```python
from build123d import *

# Parameters (mm, degrees)
BOSS_EXTRU_1_DEPTH      = 5
ENL_V_MAT_EXTRU_1_DEPTH = 3
ESQUISSE3_W             = 33.2
ESQUISSE3_H             = 3
ENL_V_MAT_EXTRU_2_DEPTH = 3
ESQUISSE4_W             = 5
ESQUISSE4_H             = 1
BOSS_EXTRU_2_DEPTH      = 0.48904
ESQUISSE5_W             = 5
ESQUISSE5_H             = 1
BOSS_EXTRU_3_DEPTH      = 0.48904
ESQUISSE6_W             = 5
ESQUISSE6_H             = 1
BOSS_EXTRU_4_DEPTH      = 0.48904


with BuildPart() as part:
    # Esquisse1 → Boss.-Extru.1 (new body)
    with BuildSketch(Plane(origin=(0, 0, 0), x_dir=(1, 0, 0), z_dir=(0, 1, 0))):
        with BuildLine():
            Line((2, 0), (36.2, 0))
            ThreePointArc((36.2, 0), (37.614213562, 0.585786438), (38.2, 2))
            Line((38.2, 2), (38.2, 25))
            ThreePointArc((38.2, 25), (37.614213562, 26.414213562), (36.2, 27))
            Line((36.2, 27), (2, 27))
            ThreePointArc((2, 27), (0.585786438, 26.414213562), (0, 25))
            Line((0, 25), (0, 2))
            ThreePointArc((0, 2), (0.585786438, 0.585786438), (2, 0))
        make_face()
    extrude(amount=BOSS_EXTRU_1_DEPTH)

    # Esquisse2 → Enlèv. mat.-Extru.1 (cut)
    with BuildSketch(Plane(origin=(0, 5, 0), x_dir=(1, 0, 0), z_dir=(0, 1, 0))):
        with BuildLine():
            Line((37.2, 2), (37.2, 25))
            ThreePointArc((37.2, 25), (36.907106781, 25.707106781), (36.2, 26))
            Line((36.2, 26), (2, 26))
            ThreePointArc((2, 26), (1.292893219, 25.707106781), (1, 25))
            Line((1, 25), (1, 2))
            ThreePointArc((1, 2), (1.292893219, 1.292893219), (2, 1))
            Line((2, 1), (36.2, 1))
            ThreePointArc((36.2, 1), (36.907106781, 1.292893219), (37.2, 2))
        make_face()
    extrude(amount=-ENL_V_MAT_EXTRU_1_DEPTH, mode=Mode.SUBTRACT)

    # Esquisse3 → Enlèv. mat.-Extru.2 (cut)
    with BuildSketch(Plane.XY):
        with Locations((19.1, 3.5)):
            Rectangle(ESQUISSE3_W, ESQUISSE3_H)
    extrude(amount=-ENL_V_MAT_EXTRU_2_DEPTH, mode=Mode.SUBTRACT)

    # Esquisse4 → Boss.-Extru.2 (add)
    with BuildSketch(Plane(origin=(1, 0, 0), x_dir=(0, 0, -1), z_dir=(1, 0, 0))):
        with Locations((13.5, 4.25)):
            Rectangle(ESQUISSE4_W, ESQUISSE4_H)
    extrude(amount=BOSS_EXTRU_2_DEPTH)

    # Esquisse5 → Boss.-Extru.3 (add)
    with BuildSketch(Plane.ZY.offset(-37.2)):
        with Locations((-13.5, 4.25)):
            Rectangle(ESQUISSE5_W, ESQUISSE5_H)
    extrude(amount=BOSS_EXTRU_3_DEPTH)

    # Esquisse6 → Boss.-Extru.4 (add)
    with BuildSketch(Plane.XY.offset(-26)):
        with Locations((9.75, 4.25)):
            Rectangle(ESQUISSE6_W, ESQUISSE6_H)
        with Locations((28.45, 4.25)):
            Rectangle(ESQUISSE6_W, ESQUISSE6_H)
    extrude(amount=BOSS_EXTRU_4_DEPTH)


solid = part.part
```
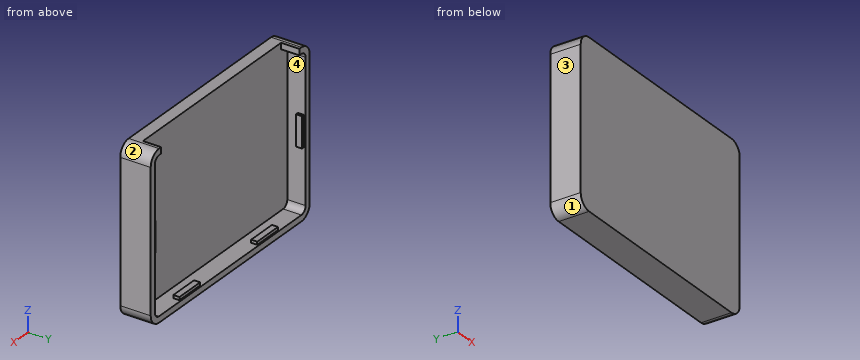
Could you check a few things on this model? Use its own coordinates, in mm. Face numbers are marked on the shaded views. Round coordinates to 2 decimals unless told otherwise and drop trailing zeros. Loops run counter-clockwise (first coordinate to the right, second up) from the corner with the lowest first, then second, coordinate; pieces in that order, holes last. Notation, with made-up numbers: (52, 76.25) - (91, 76.25) arc R28 ccw to (91, 95.25) - close; hole circle Ø11 at (-37, 1). An arc over 180 degrees is marked (long way). Answer as CSV lines item,"result".
1. I want a section at C-C on z = -5.5. List the corners of the cut face in (x, y) for me.
Filled in:
outline,"(0, 0) - (38.2, 0) - (38.2, 5) - (37.2, 5) - (37.2, 2) - (1, 2) - (1, 5) - (0, 5) - close"
2. I want a section at A-A on y = 3.35. List the corners of the cut face in (x, z) for me.
Filled in:
outline,"(0, -25) arc R2 ccw to (2, -27) - (36.2, -27) arc R2 ccw to (38.2, -25) - (38.2, -2) arc R2 ccw to (36.2, 0) - (35.7, 0) - (35.7, -1) - (36.2, -1) arc R1 cw to (37.2, -2) - (37.2, -25) arc R1 cw to (36.2, -26) - (2, -26) arc R1 cw to (1, -25) - (1, -2) arc R1 cw to (2, -1) - (2.5, -1) - (2.5, 0) - (2, 0) arc R2 ccw to (0, -2) - close"
3. We'd pull the mould along Z, two halves only. Please class the marked faces 1, 2, 3 and 4: +Z half, -Z half, draft (parallel to the pull), parting line (faces both ways), or undercut.
Filled in:
face 1,"-Z half"
face 2,"+Z half"
face 3,"draft"
face 4,"undercut"
4. For pin 1 Ø1.5 at (x, z) = (6, -13.5) entering from +Y; pin 2 Ø1 at (x, z) = (26, -15.5) entering from -Y; pin 3 Ø0.5 at (y, z) = (4, -26) entering from -X; pin 4 Ø0.5 at (x, y) = (37, 4.5) entering from -Z, each with a flat end and sliding along its axis, tell me the tip position at first contact or that it passes through.
Filled in:
pin 1,"stops at y = 2"
pin 2,"stops at y = 0"
pin 3,"stops at x = 0.15"
pin 4,"stops at z = -26.92"
5. I want a section at B-B on x = 27.5. List the corners of the cut face in (y, z) for me, then the cut area to 3 significant figures.
Filled in:
outline,"(0, -27) - (5, -27) - (5, -26) - (4.75, -26) - (4.75, -25.51) - (3.75, -25.51) - (3.75, -26) - (2, -26) - (2, 0) - (0, 0) - close"
area,"57.5 mm^2"
6. Please list where these lines run through material, in increasing order: line 1 along X through (y, z) = (4.8, -14.5); line 2 along Y through (x, z) = (18, -24.5); line 3 along Z through (x, y) = (9, 3.4). Write a range as [from, to].
Filled in:
line 1,"x = [0, 1], [37.2, 38.2]"
line 2,"y = [0, 2]"
line 3,"z = [-27, -26]"
7. I want a section at D-D on z = -11.75. List the corners of the cut face in (x, y) for me.
Filled in:
outline,"(0, 0) - (38.2, 0) - (38.2, 5) - (37.2, 5) - (37.2, 4.75) - (36.71, 4.75) - (36.71, 3.75) - (37.2, 3.75) - (37.2, 2) - (1, 2) - (1, 3.75) - (1.49, 3.75) - (1.49, 4.75) - (1, 4.75) - (1, 5) - (0, 5) - close"
